Could you check a few things on this model? Use its own coordinates, in mm. Face numbers are marked on the shaded views. A direction names the side the tool comes from. Coordinates: 2 decimals unless noted, no trailing zeros. Loops run counter-clockwise (first coordinate to the right, second up) from the corner with the lowest first, then second, coordinate; pieces in that order, holes last.
1) Imagine slicing it at C-C on z = 2.35. Please give me the cut outline in (x, y), plus the area to 3 significant figures.
2) For the marked faces 1 and 2, which set-ups out of +Z, -Z, +X, -X, +Y, -Y let a thin tool reach every point of the face, with its end or its side?
3) If I drill on line 1 along Y through (x, z) = (31, 0.7); line 2 along Y through (x, z) = (0, 2); line 3 along Z through (x, y) = (-28, 32.5), over which ranges is the centre line in solid material (lowest first)?
4) Will these pins go through, and if not, where does the flat tip stop? P1, Ø3.5, axis at x = -31.11, y = -31.11, coming from the -Z side; P2, Ø6.5, axis at x = 31.11, y = -31.11, coming from the -Z side; P3, Ø3, axis at x = -20, y = -25.5, coming from the +Z side.
5) Imagine slicing it at A-A on x = 0. Please give me the cut outline in (y, z), plus the area to 3 significant figures.
```python
from build123d import *

# Parameters (mm, degrees)
SKETCH_1_W            = 71
SKETCH_1_H            = 71
EXTRUDE_1_DEPTH       = 0.8
SKETCH_2_W            = 25
SKETCH_2_H            = 4.45
HOLE_WIZARD_M30_1_D   = 35
HOLE_WIZARD_4_0_4_1_D = 4
FILLET_1_R            = 1
FILLET_2_R            = 10
EXTRUDE_START         = -0.8
SKETCH_9_R            = 17.5
EXTRUDE_3_DEPTH       = 0.8
CUT_EXTRUDE_1_REACH   = 52.401
SKETCH_8_R            = 2


with BuildPart() as part:
    # 草图1 → 凸台-拉伸1 (new body)
    with BuildSketch(Plane.XY.offset(1)):
        Rectangle(SKETCH_1_W, SKETCH_1_H)
    extrude(amount=-EXTRUDE_1_DEPTH)

    # 草图2 → 旋转1 (revolve)
    with BuildSketch(Plane.XZ, mode=Mode.PRIVATE) as revolve_1_sk:
        with Locations((12.5, 3.225)):
            Rectangle(SKETCH_2_W, SKETCH_2_H)
    revolve(revolve_1_sk.sketch.rotate(Axis((0, 0, 5.45), (0, 0, -1)), 180), axis=Axis((0, 0, 5.45), (0, 0, -1)))

    # M30 间隙孔1 (through all)
    with Locations(Plane.XY.offset(5.45)):
        with Locations((0, 0)):
            Hole(HOLE_WIZARD_M30_1_D / 2)

    # Ø4.0 (4) 直径孔1 (through all)
    with Locations(Plane.XY.offset(1)):
        with Locations((-29, 29), (-29, -29), (29, -29), (29, 29)):
            Hole(HOLE_WIZARD_4_0_4_1_D / 2)

    # 圆角1
    fillet_1_edges = [part.edges().sort_by_distance(p)[0] for p in [
        (25, 0, 5.45),
        (17.5, 0, 5.45),
    ]]
    fillet(fillet_1_edges, radius=FILLET_1_R)

    # 圆角2
    fillet_2_edges = [part.edges().sort_by_distance(p)[0] for p in [
        (35.5, 35.5, 0.6),
        (35.5, -35.5, 0.6),
        (-35.5, -35.5, 0.6),
        (-35.5, 35.5, 0.6),
    ]]
    fillet(fillet_2_edges, radius=FILLET_2_R)

    # 草图9 → 凸台-拉伸3 (add)
    with BuildSketch(Plane.XY.offset(1).offset(EXTRUDE_START)):
        with BuildLine():
            Line((-34.5, 35.5), (34.5, 35.5))
            ThreePointArc((34.5, 35.5), (35.207106781, 35.207106781), (35.5, 34.5))
            Line((35.5, 34.5), (35.5, -34.5))
            ThreePointArc((35.5, -34.5), (35.207106781, -35.207106781), (34.5, -35.5))
            Line((34.5, -35.5), (-34.5, -35.5))
            ThreePointArc((-34.5, -35.5), (-35.207106781, -35.207106781), (-35.5, -34.5))
            Line((-35.5, -34.5), (-35.5, 34.5))
            ThreePointArc((-35.5, 34.5), (-35.207106781, 35.207106781), (-34.5, 35.5))
        make_face()
        Circle(SKETCH_9_R, mode=Mode.SUBTRACT)
    extrude(amount=EXTRUDE_3_DEPTH)

    # 草图8 → 切除-拉伸1 (cut, up to next)
    with BuildSketch(Plane.XY.offset(1), mode=Mode.PRIVATE) as cut_extrude_1_sk1:
        with Locations((-31.112698372, 31.112698372)):
            Circle(SKETCH_8_R)
    cut_extrude_1_tool1 = extrude(cut_extrude_1_sk1.sketch, amount=-CUT_EXTRUDE_1_REACH, mode=Mode.PRIVATE) & part.part
    # 草图8 → 切除-拉伸1 (cut, up to next)
    with BuildSketch(Plane.XY.offset(1), mode=Mode.PRIVATE) as cut_extrude_1_sk2:
        with Locations((31.112698372, -31.112698372)):
            Circle(SKETCH_8_R)
    cut_extrude_1_tool2 = extrude(cut_extrude_1_sk2.sketch, amount=-CUT_EXTRUDE_1_REACH, mode=Mode.PRIVATE) & part.part
    # 草图8 → 切除-拉伸1 (cut, up to next)
    with BuildSketch(Plane.XY.offset(1), mode=Mode.PRIVATE) as cut_extrude_1_sk3:
        with Locations((-31.112698372, -31.112698372)):
            Circle(SKETCH_8_R)
    cut_extrude_1_tool3 = extrude(cut_extrude_1_sk3.sketch, amount=-CUT_EXTRUDE_1_REACH, mode=Mode.PRIVATE) & part.part
    # 草图8 → 切除-拉伸1 (cut, up to next)
    with BuildSketch(Plane.XY.offset(1), mode=Mode.PRIVATE) as cut_extrude_1_sk4:
        with Locations((31.112698372, 31.112698372)):
            Circle(SKETCH_8_R)
    cut_extrude_1_tool4 = extrude(cut_extrude_1_sk4.sketch, amount=-CUT_EXTRUDE_1_REACH, mode=Mode.PRIVATE) & part.part
    add(cut_extrude_1_tool1.solids().sort_by_distance((-31.112698, 31.112698, 1))[0], mode=Mode.SUBTRACT)
    add(cut_extrude_1_tool2.solids().sort_by_distance((31.112698, -31.112698, 1))[0], mode=Mode.SUBTRACT)
    add(cut_extrude_1_tool3.solids().sort_by_distance((-31.112698, -31.112698, 1))[0], mode=Mode.SUBTRACT)
    add(cut_extrude_1_tool4.solids().sort_by_distance((31.112698, 31.112698, 1))[0], mode=Mode.SUBTRACT)


solid = part.part
```
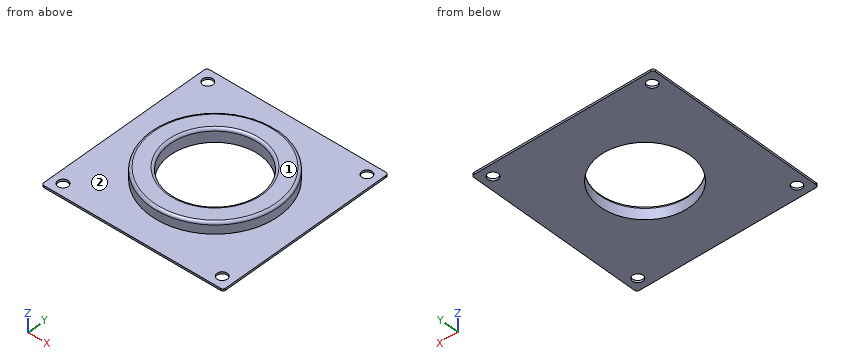
Filled in:
1. outline: circle Ø50 at (0, 0); hole circle Ø35 at (0, 0)
1. area: 1,000 mm2
2. face 1: +Z, +X, -X, +Y, -Y
2. face 2: +Z
3. line 1: y = -35.5 to -33.11, -29.12 to 29.12, 33.11 to 35.5
3. line 2: y = -25 to -17.5, 17.5 to 25
3. line 3: z = 0.2 to 1
4. P1: passes through
4. P2: stops at z = 0.2
4. P3: stops at z = 1
5. outline: (-35.5, 0.2) - (-17.5, 0.2) - (-17.5, 4.45) arc R1 ccw to (-18.5, 5.45) - (-24, 5.45) arc R1 ccw to (-25, 4.45) - (-25, 1) - (-35.5, 1) - close; (17.5, 0.2) - (35.5, 0.2) - (35.5, 1) - (25, 1) - (25, 4.45) arc R1 ccw to (24, 5.45) - (18.5, 5.45) arc R1 ccw to (17.5, 4.45) - close
5. area: 94.7 mm2
